from build123d import *

# Parameters (mm, degrees)
F0_W     = 50
F0_H     = 25
F1_DEPTH = 3
F2_R     = 6
F3_DEPTH = 3.001
F5_DEPTH = 3.001
F6_R     = 2
F7_DEPTH = 3.001
F9_DEPTH = 3.001


with BuildPart() as f1:
    # F0 (on Top) → F1 (new body)
    with BuildSketch(Plane.XY):
        Rectangle(F0_W, F0_H)
    extrude(amount=F1_DEPTH)

    # F2 (on face) → F3 (cut, through all)
    with BuildSketch(Plane.XY.offset(3)):
        Circle(F2_R)
    extrude(amount=-F3_DEPTH, mode=Mode.SUBTRACT)

    # F4 (on face) → F5 (cut, through all)
    with BuildSketch(Plane.XY.offset(3)):
        Polygon((-25, 12.5), (-25, 0), (-8, 12.5), align=None)
        Polygon((-8, -12.5), (-25, 0), (-25, -12.5), align=None)
        Polygon((25, 12.5), (8, 12.5), (25, 0), align=None)
        Polygon((25, 0), (8, -12.5), (25, -12.5), align=None)
    extrude(amount=-F5_DEPTH, mode=Mode.SUBTRACT)

    # F6 (on face) → F7 (cut, through all)
    with BuildSketch(Plane.XY.offset(3)):
        with Locations((-15, 0)):
            Circle(F6_R)
        with Locations((15, 0)):
            Circle(F6_R)
    extrude(amount=-F7_DEPTH, mode=Mode.SUBTRACT)

    # F8 (on face) → F9 (cut, through all)
    with BuildSketch(Plane.XY.offset(3)):
        Polygon((-21.6, -2.5), (-21.6, 2.5), (-25, 0), align=None)
        Polygon((25, 0), (21.6, 2.5), (21.6, -2.5), align=None)
    extrude(amount=-F9_DEPTH, mode=Mode.SUBTRACT)


solid = f1.part
Can you work these out from the model? Positions are in its coordinate system, mm. Round coordinates to 2 decimals unless told otherwise and drop trailing zeros. Write each loop counter-clockwise with the first axis right and the second up, starting at its lowest first coordinate (ties: lowest second). Pieces come first, ordered by that corner, then holes. Notation, with made-up numbers: (-11, -12) -> (9, -12) arc R15 cw to (9, 6) -> close; hole circle Ø1 at (-25, 53). An arc over 180 degrees is marked (long way). One line per question, with ' | ' between items. Start each with the question number.
1) Suppose I cut it at A-A on y = 0. Write out the boundary of the cut face in (x, z).
2) Suppose I cut it at C-C on z = 2.2. Write out the boundary of the cut face in (x, y).
3) I'm going to push a flat-ended pin straight in: P1, Ø1, axis at x = -9.5, z = 2, coming from the -Y side. Where does the tip first touch, or does it pass through?
4) If we mould it in two halves opening along Y, with no side actions, what happens to faces 1 (the cylindrical face through (-6, 0, 2)), 2 (the flat face through (21.6, 0, 2)), 3 (the cylindrical face through (-16.6, -1.2, 1.5)), 4 (the flat face through (-14.705, -7.57, 1.521))? For each: released by +Y, released by -Y, zero draft, split by the parting line, or undercut.
5) Suppose I cut it at D-D on y = 3.75. Write out the boundary of the cut face in (x, z).
6) Suppose I cut it at B-B on x = 0. Write out the boundary of the cut face in (y, z), then the cut area to 3 significant figures.
7) I need wall thicknesses on line 1 (Y direction, x = 0, z = 1.8); line 2 (X direction, y = 4, z = 0.75); line 3 (X direction, y = 3.25, z = 1.55). Which ranges of each line are inside material? Lowest first, please. Write a range as [from, to].
Return value:
1) outline: (-21.6, 0) -> (-17, 0) -> (-17, 3) -> (-21.6, 3) -> close; (-13, 0) -> (-6, 0) -> (-6, 3) -> (-13, 3) -> close; (6, 0) -> (13, 0) -> (13, 3) -> (6, 3) -> close; (17, 0) -> (21.6, 0) -> (21.6, 3) -> (17, 3) -> close
2) outline: (-21.6, -2.5) -> (-8, -12.5) -> (8, -12.5) -> (21.6, -2.5) -> (21.6, 2.5) -> (8, 12.5) -> (-8, 12.5) -> (-21.6, 2.5) -> close; hole circle Ø4 at (-15, 0); hole circle Ø12 at (0, 0); hole circle Ø4 at (15, 0)
3) P1: stops at y = -11.76
4) face 1: undercut | face 2: zero draft | face 3: undercut | face 4: released by -Y
5) outline: (-19.9, 0) -> (-4.68, 0) -> (-4.68, 3) -> (-19.9, 3) -> close; (4.68, 0) -> (19.9, 0) -> (19.9, 3) -> (4.68, 3) -> close
6) outline: (-12.5, 0) -> (-6, 0) -> (-6, 3) -> (-12.5, 3) -> close; (6, 0) -> (12.5, 0) -> (12.5, 3) -> (6, 3) -> close | area: 39.0 mm2
7) line 1: y = [-12.5, -6], [6, 12.5] | line 2: x = [-19.56, -4.47], [4.47, 19.56] | line 3: x = [-20.58, -5.04], [5.04, 20.58]
